Here's the drawing with two shaded views (mm, measured from the low corner). I have some questions. A direction names the side the tool comes from. Give positions to 0.01 mm unless a question says otherwise; leave off trailing zeros. Loops run counter-clockwise (first coordinate to the right, second up) from the corner with the lowest first, then second, coordinate; pieces in that order, holes last.
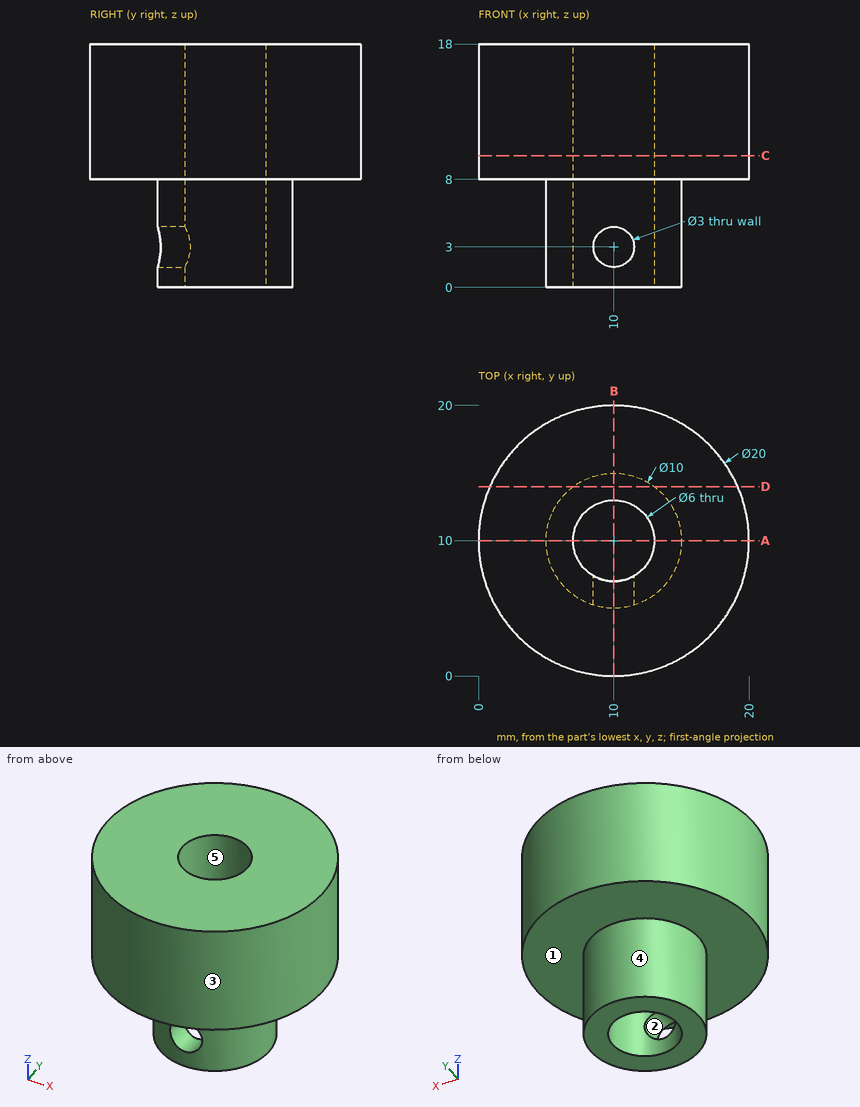
(1) Thinking about a two-plate mould opening in X: for the marked faces 1, 2 and 3, which applies, pulls with the +X half, pulls with the -X half, needs draft (parallel to the pull), parting line crosses it, or undercut?
Returned:
face 1: needs draft
face 2: undercut
face 3: parting line crosses it
(2) Suppose I cut it at D-D on y = 14. List the corners of the cut face in (x, z) for me, plus the area to 3 significant figures.
Returned:
outline: (0.83, 8) - (7, 8) - (7, 0) - (13, 0) - (13, 8) - (19.17, 8) - (19.17, 18) - (0.83, 18) - close
area: 231 mm2
(3) Suppose I cut it at C-C on z = 9.75. List the corners of the cut face in (x, y) for me.
Returned:
outline: circle Ø20 at (10, 10); hole circle Ø6 at (10, 10)
(4) Will these pins go through, and if not, where does the flat tip stop? P1, Ø5.5, axis at x = 10, y = 10, coming from the +Z side; P2, Ø2, axis at x = 7.5, z = 10, coming from the +Y side; P3, Ø1.5, axis at x = 14, y = 2.5, coming from the -Z side; P4, Ø5, axis at x = 10, z = 3, coming from the +Y side.
Returned:
P1: passes through
P2: stops at y = 19.89
P3: stops at z = 8
P4: stops at y = 15
(5) Suppose I cut it at B-B on x = 10. List the corners of the cut face in (y, z) for me.
Returned:
outline: (0, 8) - (5, 8) - (5, 4.5) - (7, 4.5) - (7, 18) - (0, 18) - close; (5, 0) - (7, 0) - (7, 1.5) - (5, 1.5) - close; (13, 0) - (15, 0) - (15, 8) - (20, 8) - (20, 18) - (13, 18) - close
(6) Which directions (+Z, -Z, +X, -X, +Y, -Y) give clear straight access to the entire face, cutting with the end or side of a thin tool? Please do the marked faces 4 and 5.
Returned:
face 4: -Z
face 5: +Z, -Z
(7) Suppose I cut it at A-A on y = 10. List the corners of the cut face in (x, z) for me.
Returned:
outline: (0, 8) - (5, 8) - (5, 0) - (7, 0) - (7, 18) - (0, 18) - close; (13, 0) - (15, 0) - (15, 8) - (20, 8) - (20, 18) - (13, 18) - close
(8) Please list where these lines run through material, in increasing order: probe 1 along Z at (x, y) = (10, 6.55); probe 2 along Y at (x, z) = (10, 14.25); probe 3 along Z at (x, y) = (15.25, 4.5).
Returned:
probe 1: z = 0 to 1.5, 4.5 to 18
probe 2: y = 0 to 7, 13 to 20
probe 3: z = 8 to 18
